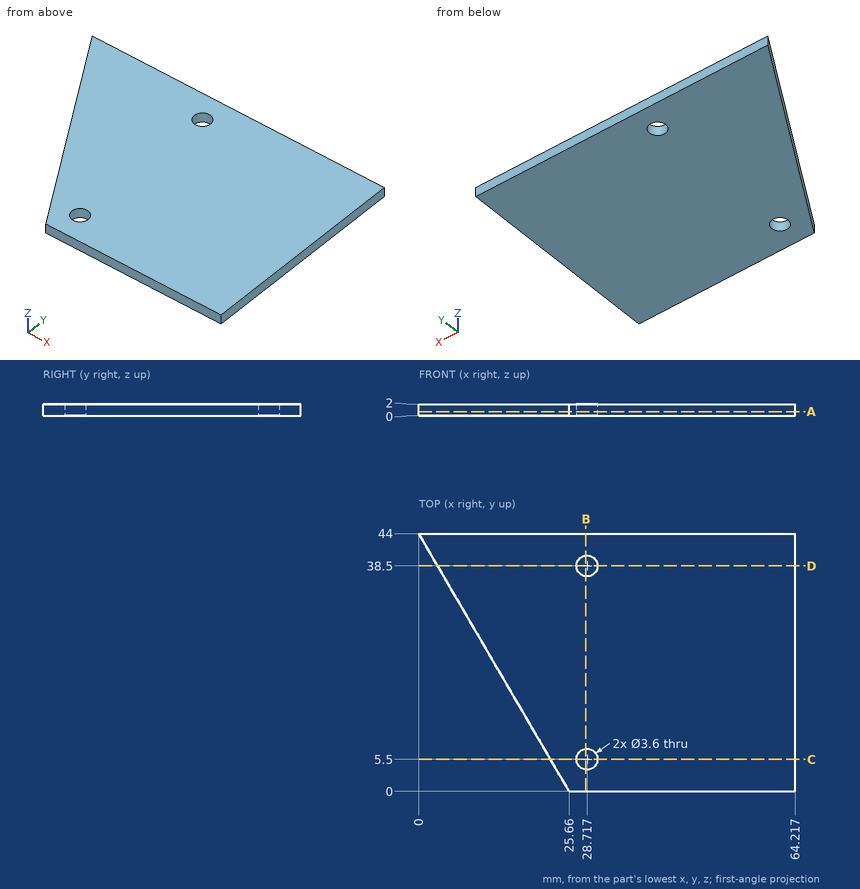
Could you check a few things on this drawing? It's one solid part, dimensions in mm from its lowest x, y, z. Give positions to 0.01 mm unless a question says otherwise; leave off trailing zeros. Loops run counter-clockwise (first coordinate to the right, second up) from the corner with the lowest first, then second, coordinate; pieces in that order, holes last. Notation, with made-up numbers: M 43.5,16.5 L 51.5,16.5 A21 ccw 51.5,20.5 Z; hole C 60.25,-31.75 d2. An arc over 180 degrees is marked long. Answer as a JSON object with one key per item and string values.
Q1. Suppose I cut it at D-D, the plane y = 38.5. List the corners of the cut face in (x, z) for me.
Values found:
{"outline": "M 3.21,0 L 26.92,0 L 26.92,2 L 3.21,2 Z; M 30.52,0 L 64.22,0 L 64.22,2 L 30.52,2 Z"}
Q2. For P1, Ø1, axis at x = 11, z = 0.5, coming from the -Y side, with a flat end and sliding along its axis, tell me the tip position at first contact or that it passes through.
Values found:
{"P1": "stops at y = 24.28"}
Q3. Suppose I cut it at B-B, the plane x = 28.5. List the corners of the cut face in (y, z) for me.
Values found:
{"outline": "M 0,0 L 3.71,0 L 3.71,2 L 0,2 Z; M 7.29,0 L 36.71,0 L 36.71,2 L 7.29,2 Z; M 40.29,0 L 44,0 L 44,2 L 40.29,2 Z"}
Q4. If I drill on probe 1 along X at (y, z) = (6, 1.3) (1 decimal); probe 2 along X at (y, z) = (4.5, 1.05) (1 decimal); probe 3 along Y at (x, z) = (25.5, 0.9) (1 decimal), over which ranges is the centre line in solid material (lowest first)? Write a range as [from, to].
Values found:
{"probe 1": "x = [22.2, 27], [30.4, 64.2]", "probe 2": "x = [23, 27.2], [30.2, 64.2]", "probe 3": "y = [0.3, 44]"}
Q5. Suppose I cut it at A-A, the plane z = 0.7. List the corners of the cut face in (x, y) for me.
Values found:
{"outline": "M 0,44 L 25.66,0 L 64.22,0 L 64.22,44 Z; hole C 28.72,5.5 d3.6; hole C 28.72,38.5 d3.6"}
Q6. Suppose I cut it at C-C, the plane y = 5.5. List the corners of the cut face in (x, z) for me.
Values found:
{"outline": "M 22.45,0 L 26.92,0 L 26.92,2 L 22.45,2 Z; M 30.52,0 L 64.22,0 L 64.22,2 L 30.52,2 Z"}
